```python
from build123d import *

# Parameters (mm, degrees)
SKETCH3_W           = 7.785
SKETCH3_H           = 7.785
SKETCH3_W_2         = 3.785
SKETCH3_H_2         = 3.785
BOSS_EXTRUDE1_DEPTH = 4
SKETCH4_R           = 12.5
BOSS_EXTRUDE2_DEPTH = 6
SKETCH5_R           = 13.5
BOSS_EXTRUDE3_DEPTH = 1
FILLET1_R           = 1


with BuildPart() as part:
    # Sketch3 → Boss-Extrude1 (new body)
    with BuildSketch(Plane(origin=(0, 0, 0), x_dir=(1, 0, 0), z_dir=(0, 1, 0))):
        Rectangle(SKETCH3_W, SKETCH3_H)
        Rectangle(SKETCH3_W_2, SKETCH3_H_2, mode=Mode.SUBTRACT)
    extrude(amount=BOSS_EXTRUDE1_DEPTH)

    # Sketch4 → Boss-Extrude2 (add)
    with BuildSketch(Plane(origin=(0, 4, 0), x_dir=(1, 0, 0), z_dir=(0, 1, 0))):
        with Locations(Location((0, 0, 0), (0, 0, 270))):
            Circle(SKETCH4_R)
    extrude(amount=BOSS_EXTRUDE2_DEPTH)

    # Sketch5 → Boss-Extrude3 (add)
    with BuildSketch(Plane.XZ.offset(-4)):
        with Locations(Location((0, 0, 0), (0, 0, 270))):
            Circle(SKETCH5_R)
    extrude(amount=-BOSS_EXTRUDE3_DEPTH)

    # Fillet1
    fillet1_edges = [part.edges().sort_by_distance(p)[0] for p in [
        (3.8925, 2, 3.8925),
        (-3.8925, 2, 3.8925),
        (-3.8925, 2, -3.8925),
        (3.8925, 2, -3.8925),
    ]]
    fillet(fillet1_edges, radius=FILLET1_R)


solid = part.part
```
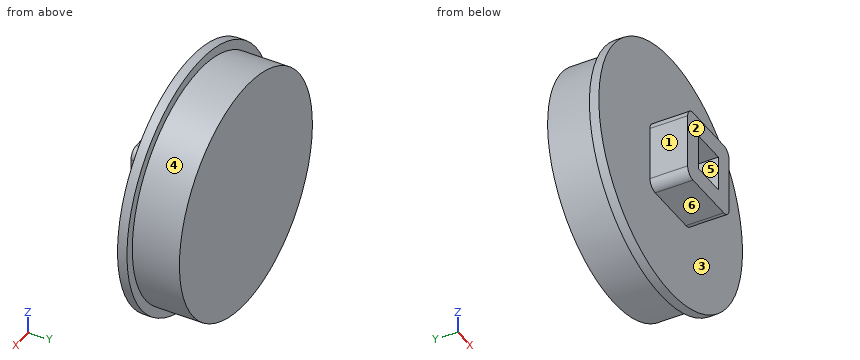
Verification items for the finished model (mm, model axes). Face numbers are marked on the shaded views. A direction names the side the tool comes from. Round coordinates to 2 decimals unless told otherwise and drop trailing zeros. Write each loop counter-clockwise with the first axis right and the second up, starting at its lowest first coordinate (ties: lowest second). Pieces come first, ordered by that corner, then holes. Notation, with made-up numbers: (-23.75, 54.5) -> (20.25, 54.5) arc R18 ccw to (20.25, 64.5) -> close; hole circle Ø2 at (40.5, 44.5). An arc over 180 degrees is marked (long way). Write each question's results on one line, items separated by ' | '. Start each with the question number.
1. Cross-section at C-C (x = 0). Enter the section's corners in (y, z), then the cut area to 3 significant figures.
2. Set-up check for the marked faces 1, 2 and 3: record each of +Z, -Z, +X, -X, +Y, -Y from which the full face is reachable in a straight line by a thin tool's end or side.
3. Cross-section at A-A (z = 0). Enter the section's corners in (x, y), then the cut area to 3 significant figures.
4. Material ranges on probe 1 along Y at (x, z) = (1, -7); probe 2 along Y at (x, z) = (-12, 3.75); probe 3 along Z at (x, y) = (0.25, 6.5), recorded low to high. Write a range as from..to.
5. Depth check by flat-ended pin: P1, Ø4, axis at y = 1.5, z = 0.5, coming from the -X side; P2, Ø3, axis at x = 0.5, y = 2, coming from the +Z side; P3, Ø1.5, axis at y = 8.5, z = -9, coming from the +X side; P4, Ø4, axis at x = -0.5, z = -0.5, coming from the -Y side. Enter the tip coordinate at first touch or a pass-through.
6. Cross-section at D-D (y = 6). Enter the section's corners in (x, z).
7. Draft check along Z on the marked faces 4, 5 and 6. Enter one of: +Z half, -Z half, draft (parallel to the pull), parting line (faces both ways), or undercut.
8. Cross-section at B-B (y = 2). Enter the section's corners in (x, z), then the cut area to 3 significant figures.
Solutions:
1) outline: (0, -3.89) -> (4, -3.89) -> (4, -13.5) -> (5, -13.5) -> (5, -12.5) -> (10, -12.5) -> (10, 12.5) -> (5, 12.5) -> (5, 13.5) -> (4, 13.5) -> (4, 3.89) -> (0, 3.89) -> (0, 1.89) -> (4, 1.89) -> (4, -1.89) -> (0, -1.89) -> close | area: 168 mm2
2) face 1: +Z, -Z, -X, -Y | face 2: +Z, -Z, +X, -X, -Y | face 3: -Y
3) outline: (-13.5, 4) -> (-3.89, 4) -> (-3.89, 0) -> (-1.89, 0) -> (-1.89, 4) -> (1.89, 4) -> (1.89, 0) -> (3.89, 0) -> (3.89, 4) -> (13.5, 4) -> (13.5, 5) -> (12.5, 5) -> (12.5, 10) -> (-12.5, 10) -> (-12.5, 5) -> (-13.5, 5) -> close | area: 168 mm2
4) probe 1: y = 4..10 | probe 2: y = 4..5 | probe 3: z = -12.5..12.5
5) P1: stops at x = -3.89 | P2: stops at z = 3.89 | P3: stops at x = 9.39 | P4: stops at y = 0
6) outline: circle Ø25 at (0, 0)
7) face 4: parting line | face 5: undercut | face 6: -Z half
8) outline: (-3.89, -2.89) arc R1 ccw to (-2.89, -3.89) -> (2.89, -3.89) arc R1 ccw to (3.89, -2.89) -> (3.89, 2.89) arc R1 ccw to (2.89, 3.89) -> (-2.89, 3.89) arc R1 ccw to (-3.89, 2.89) -> close; hole (-1.89, -1.89) -> (1.89, -1.89) -> (1.89, 1.89) -> (-1.89, 1.89) -> close | area: 45.4 mm2
